```python
from build123d import *

# Parameters (mm, degrees)
SKETCH1_R           = 12.5
SKETCH1_R_2         = 6.75
BOSS_EXTRUDE1_DEPTH = 2
SKETCH1_3_R         = 6.75
SKETCH1_3_R_2       = 5.75
BOSS_EXTRUDE2_DEPTH = 120
SKETCH1_4_R         = 5.75
CUT_EXTRUDE1_DEPTH  = 115
SKETCH2_W           = 5.5
SKETCH2_H           = 5.53257791
CUT_EXTRUDE3_DEPTH  = 80


with BuildPart() as part:
    # Sketch1 → Boss-Extrude1 (new body)
    with BuildSketch(Plane.XY):
        Circle(SKETCH1_R)
        Circle(SKETCH1_R_2, mode=Mode.SUBTRACT)
    extrude(amount=BOSS_EXTRUDE1_DEPTH)

    # Sketch1_3 → Boss-Extrude2 (add)
    # profile 1 of 2: a face of its own
    with BuildSketch(Plane.XY):
        Circle(SKETCH1_3_R)
        Circle(SKETCH1_3_R_2, mode=Mode.SUBTRACT)
    # profile 2 of 2: a face of its own
    with BuildSketch(Plane.XY):
        Circle(SKETCH1_3_R_2)
    extrude(amount=BOSS_EXTRUDE2_DEPTH)

    # Sketch1_4 → Cut-Extrude1 (cut)
    with BuildSketch(Plane.XY):
        Circle(SKETCH1_4_R)
    extrude(amount=CUT_EXTRUDE1_DEPTH, mode=Mode.SUBTRACT)

    # Sketch2 → Cut-Extrude3 (cut)
    with BuildSketch(Plane.XY.offset(10)):
        with Locations((0, -6.75)):
            Rectangle(SKETCH2_W, SKETCH2_H)
    extrude(amount=CUT_EXTRUDE3_DEPTH, mode=Mode.SUBTRACT)


solid = part.part
```
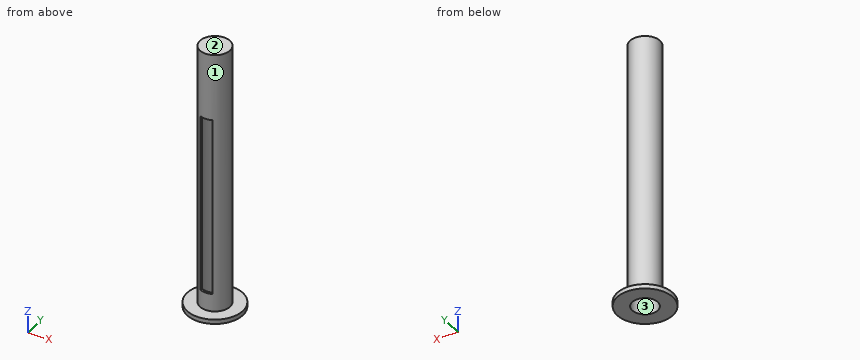
Read the model definition and answer for the solid it produces. Units are mm, in the model's axes. Face numbers are marked on the shaded views. Round coordinates to 2 decimals unless told otherwise and drop trailing zeros. Write each loop counter-clockwise with the first axis right and the second up, starting at its lowest first coordinate (ties: lowest second). Pieces come first, ordered by that corner, then holes. Notation, with made-up numbers: (58.25, 34) -> (66.25, 34) arc R14 ccw to (66.25, 39) -> close; hole circle Ø4 at (-20.75, 24.5). An arc over 180 degrees is marked (long way). Answer in a Markdown table with one row per item. Add a question column.
1) Find section B-B, the plane y = 0. Determine the outline of the cut face in (x, z), and give its area (4 significant figures).
2) Find section C-C, the plane z = 110. Determine the outline of the cut face in (x, y).
3) Find section A-A, the plane x = 0. Determine the outline of the cut face in (y, z), and give its area (4 significant figures).
4) Determine the mould class of the marked faces 1, 2 and 3 for opening direction Y: pulls with the +Y half, pulls with the -Y half, needs draft (parallel to the pull), parting line crosses it, or undercut.
5) Find section D-D, the plane z = 59.5. Determine the outline of the cut face in (x, y), and give its area (3 significant figures).
6) Given P1, Ø3, axis at y = 2.5, z = 37.5, coming from the -X side; P2, Ø2, axis at x = -8, y = -3, coming from the -Z side; P3, Ø1.2, axis at y = -6, z = 34.5, coming from the -X side; P4, Ø6, axis at x = -4, y = -9, coming from the +Z side, each flat-ended and moving along its own axis, determine where each tip first touches the part or whether it passes through.
7) Consider line 1 (X direction, y = -0.5, z = 7); line 2 (Z direction, x = -6.25, y = -8.5); line 3 (Y direction, x = -5, z = 19.5). Determine where each line is inside the solid, lowest interval first.
Findings below:
| question | item | result |
|---|---|---|
| 1 | outline | (-12.5, 0) -> (-5.75, 0) -> (-5.75, 115) -> (5.75, 115) -> (5.75, 0) -> (12.5, 0) -> (12.5, 2) -> (6.75, 2) -> (6.75, 120) -> (-6.75, 120) -> (-6.75, 2) -> (-12.5, 2) -> close |
| 1 | area | 320.5 mm² |
| 2 | outline | circle Ø13.5 at (0, 0); hole circle Ø11.5 at (0, 0) |
| 3 | outline | (-12.5, 0) -> (-5.75, 0) -> (-5.75, 10) -> (-6.75, 10) -> (-6.75, 2) -> (-12.5, 2) -> close; (-6.75, 90) -> (-5.75, 90) -> (-5.75, 115) -> (5.75, 115) -> (5.75, 0) -> (12.5, 0) -> (12.5, 2) -> (6.75, 2) -> (6.75, 120) -> (-6.75, 120) -> close |
| 3 | area | 240.5 mm² |
| 4 | face 1 | parting line crosses it |
| 4 | face 2 | needs draft |
| 4 | face 3 | undercut |
| 5 | outline | (-2.75, -6.16) -> (-2.75, -5.05) arc R5.75 cw (long way) to (2.75, -5.05) -> (2.75, -6.16) arc R6.75 ccw (long way) to start |
| 5 | area | 33.6 mm² |
| 6 | P1 | x = -6.68 |
| 6 | P2 | z = 0 |
| 6 | P3 | x = -4.05 |
| 6 | P4 | z = 2 |
| 7 | line 1 | -6.73 to -5.73, 5.73 to 6.73 |
| 7 | line 2 | 0 to 2 |
| 7 | line 3 | -4.53 to -2.84, 2.84 to 4.53 |
